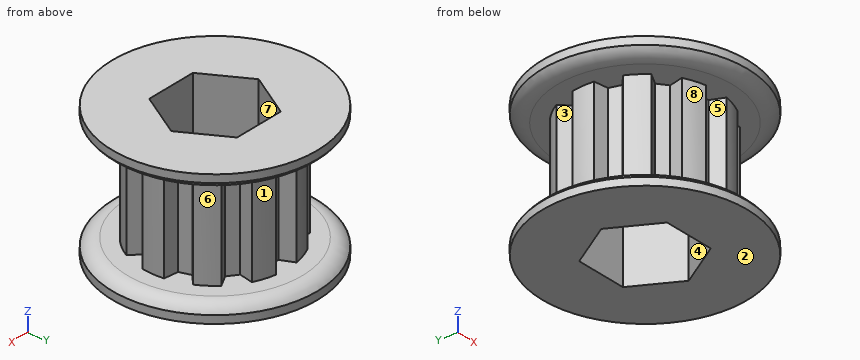
```python
from build123d import *

# Parameters (mm, degrees)
CUT_EXTRUDE1_START = 2.2987
CUT_EXTRUDE1_DEPTH = 10.922
CIRPATTERN1_COUNT  = 10
CUT_EXTRUDE2_DEPTH = 25.654


with BuildPart() as part:
    # Sketch2 → Revolve1 (revolve)
    with BuildSketch(Plane(origin=(0, 0, 0), x_dir=(0, 0, -1), z_dir=(1, 0, 0)), mode=Mode.PRIVATE) as revolve1_sk:
        with BuildLine():
            Line((-3.9878, 2.5), (10.3124, 2.5))
            Line((10.3124, 2.5), (10.3124, 11.1125))
            Line((10.3124, 11.1125), (9.46785, 11.1125))
            ThreePointArc((9.46785, 11.1125), (8.846862309, 10.395787163), (8.6233, 9.4742))
            Line((8.6233, 9.4742), (8.6233, 7.8359))
            Line((8.6233, 7.8359), (-2.2987, 7.8359))
            Line((-2.2987, 7.8359), (-2.2987, 9.4742))
            ThreePointArc((-2.2987, 9.4742), (-2.522262309, 10.395787163), (-3.14325, 11.1125))
            Line((-3.14325, 11.1125), (-3.9878, 11.1125))
            Line((-3.9878, 11.1125), (-3.9878, 2.5))
        make_face()
    revolve(revolve1_sk.sketch.rotate(Axis((0, 0, 10.3124), (0, 0, -1)), 90), axis=Axis((0, 0, 10.3124), (0, 0, -1)))

    # Sketch3 → Cut-Extrude1 (cut)
    with BuildSketch(Plane.XY.offset(CUT_EXTRUDE1_START)):
        with BuildLine():
            Line((-0.635, 6.329348022), (0.635, 6.329348022))
            Line((0.635, 6.329348022), (1.287830721, 7.729348022))
            ThreePointArc((1.287830721, 7.729348022), (0, 7.8359), (-1.287830721, 7.729348022))
            Line((-1.287830721, 7.729348022), (-0.635, 6.329348022))
        make_face()
    cut_extrude1 = extrude(amount=-CUT_EXTRUDE1_DEPTH, mode=Mode.SUBTRACT)

    # CirPattern1: Cut-Extrude1 ×10 about axis
    cirpattern1_axis = Axis((0, 0, 0), (0, 0, 1))
    for i in range(1, CIRPATTERN1_COUNT):
        add(cut_extrude1.rotate(cirpattern1_axis, i * 360 / CIRPATTERN1_COUNT), mode=Mode.SUBTRACT)

    # Sketch6 → Cut-Extrude2 (cut)
    with BuildSketch(Plane(origin=(0, 0, -10.3124), x_dir=(-1, 0, 0), z_dir=(0, 0, -1))):
        Polygon((5.499261314, 0), (2.749630657, 4.7625), (-2.749630657, 4.7625), (-5.499261314, 0), (-2.749630657, -4.7625), (2.749630657, -4.7625), align=None)
    extrude(amount=-CUT_EXTRUDE2_DEPTH, mode=Mode.SUBTRACT)


solid = part.part
```
Can you work these out from the model? Positions are in its coordinate system, mm. Face numbers are marked on the shaded views. A direction names the side the tool comes from. Coordinates: 2 decimals unless noted, no trailing zeros. Loops run counter-clockwise (first coordinate to the right, second up) from the corner with the lowest first, then second, coordinate; pieces in that order, holes last. Notation, with made-up numbers: (82.25, 29) - (95.25, 29) arc R9 cw to (95.25, 33) - close; hole circle Ø7 at (47, -32.5). An arc over 180 degrees is marked (long way). Use a Markdown table: item, result.
Item 1: We'd pull the mould along X, two halves only. Please class the marked faces 1, 2, 3 and 4: released by +X, released by -X, zero draft, split by the parting line, or undercut.
Numbers:
| item | result |
|---|---|
| face 1 | released by +X |
| face 2 | zero draft |
| face 3 | released by -X |
| face 4 | undercut |
Item 2: I want a section at B-B on z = 2.75. Please give me the cut outline in (x, y).
Numbers:
| item | result |
|---|---|
| outline | circle Ø21.49 at (0, 0); hole (-5.5, 0) - (-2.75, -4.76) - (2.75, -4.76) - (5.5, 0) - (2.75, 4.76) - (-2.75, 4.76) - close |
Item 3: If I drill on probe 1 along Z at (x, y) = (4.5, 5.5); probe 2 along Y at (x, z) = (6.75, -6); probe 3 along X at (y, z) = (-3.5, -8.5), over which ranges is the centre line in solid material (lowest first)? Write a range as from..to.
Numbers:
| item | result |
|---|---|
| probe 1 | z = -10.31..-8.62, 2.3..3.99 |
| probe 2 | y = -3.98..-3.42, -1.29..1.29, 3.42..3.98 |
| probe 3 | x = -6.83..-3.48, 3.48..6.83 |
Item 4: For the marked faces 5, 6, 7 and 8, which set-ups out of +Z, -Z, +X, -X, +Y, -Y let a thin tool reach every point of the face, with its end or its side?
Numbers:
| item | result |
|---|---|
| face 5 | -Y |
| face 6 | +X, +Y |
| face 7 | +Z, -Z |
| face 8 | -X, -Y |
Item 5: Will these pins go through, and if not, where does the flat tip stop? pin 1 (1.5 mm diameter, centred on y = 7.5, z = -5, fed in from +X); pin 2 (1.6 mm diameter, centred on x = 0, z = 0, fed in from -Y); pin 3 (2.5 mm diameter, centred on x = 1, z = -5, fed in from +Y).
Numbers:
| item | result |
|---|---|
| pin 1 | stops at x = 3.5 |
| pin 2 | stops at y = -6.68 |
| pin 3 | stops at y = 7.73 |
Item 6: I want a section at A-A on x = 0. Please give me the cut outline in (y, z), and give its area (3 significant figures).
Numbers:
| item | result |
|---|---|
| outline | (-11.11, -10.31) - (-4.76, -10.31) - (-4.76, 3.99) - (-11.11, 3.99) - (-11.11, 3.14) arc R2.01 ccw to (-9.47, 2.3) - (-6.33, 2.3) - (-6.33, -8.62) - (-9.47, -8.62) arc R2.01 ccw to (-11.11, -9.47) - close; (4.76, -10.31) - (11.11, -10.31) - (11.11, -9.47) arc R2.01 ccw to (9.47, -8.62) - (6.33, -8.62) - (6.33, 2.3) - (9.47, 2.3) arc R2.01 ccw to (11.11, 3.14) - (11.11, 3.99) - (4.76, 3.99) - close |
| area | 75.5 mm2 |
